Autodesk Inventor part; units mm, degrees
ref_plane "YZ Plane" through (0, 0, 0) normal (1, 0, 0) x (0, 1, 0)
ref_plane "XZ Plane" through (0, 0, 0) normal (0, 1, 0) x (-1, 0, 0)
ref_plane "XY Plane" through (0, 0, 0) normal (0, 0, 1) x (1, 0, 0)
sketch "Esquisse1" plane through (0, 0, 0) normal (0, 0, 1) x (1, 0, 0)
  circle A0 centre (28.6, 24.9) radius 1.5
  circle A1 centre (28.6, -24.78) radius 1.5
  circle A2 centre (-28.75, 24.9) radius 1.5
  circle A3 centre (-28.75, -24.78) radius 1.5
  line L0 (31.1, 27.4) -> (-31.25, 27.4)
  line L1 (-31.25, 27.4) -> (-31.25, -27.28)
  line L2 (-31.25, -27.28) -> (31.1, -27.28)
  line L3 (31.1, -27.28) -> (31.1, 27.4)
  line L4 (-7.575, 16) -> (-0.075, 16)
  line L5 (-0.075, 16) -> (7.425, 16)
  line L6 (7.425, 16) -> (7.425, 10)
  line L7 (7.425, 10) -> (-0.075, 10)
  line L8 (-0.075, 10) -> (-7.575, 10)
  line L9 (-7.575, 10) -> (-7.575, 16)
  line L10 (-0.075, 37.051) -> (-0.075, -38.1524) construction
  line L11 (34.7968, 0.06) -> (-21.7073, 0.06) construction
  line L12 (-7.575, -15.88) -> (-0.075, -15.88)
  line L13 (-0.075, -15.88) -> (7.425, -15.88)
  line L14 (7.425, -15.88) -> (7.425, -9.88)
  line L15 (7.425, -9.88) -> (-0.075, -9.88)
  line L16 (-0.075, -9.88) -> (-7.575, -9.88)
  line L17 (-7.575, -9.88) -> (-7.575, -15.88)
  line L18 (-0.075, -36.931) -> (-0.075, 38.2724) construction
  point P0 (0, 0)
  point P1 (-0.075, 27.4)
  point P2 (31.1, 0.06)
  dimension "d0" = 7.5
  dimension "d1" = 16
  dimension "d2" = 6
extrude "Extrusion1" add sketch "Esquisse1" along normal blind 6
equation "\"d0\" = 0.5 * L_attache_carte"
equation "\"d2\" = epaisseur"
equation "\"d3\" = epaisseur"
equation "\"epaisseur\" = 6"
equation "\"ecartement\" = 25"
equation "\"dvis\" = 3"
equation "\"largeur\" = 32"
equation "\"L_attache_carte\" = 15"
equation "\"marge_attache_carte\" = 5"
equation "\"L_cubi\" = 81.6"
equation "\"taille_trou\" = 7"
equation "\"L_moteur\" = 28.3"
equation "\"marge_trou\" = 2"
equation "\"largeur_cubi\" = 81.6"
equation "\"H_cubi\" = 81.6"
equation "\"epaisseur_wheel\" = 9"
equation "\"H_nez\" = 25"
equation "\"chanfrein\" = 0.5"
equation "\"H_trou_int\" = 0.2"
equation "\"L_trou_int\" = 1"
equation "\"pos_trou_int_1\" = 0.7"
equation "\"pos_trou_int_2\" = 3"
equation "\"epaisseur_metabois\" = 3"
equation "\"L_metabois\" = 8.2"
equation "\"epaisseur_modules\" = 6"
properties part number "support_card"
Verification items for the finished model (mm, model axes). A direction names the side the tool comes from. Give positions to 0.01 mm unless a question says otherwise; leave off trailing zeros. Write each loop counter-clockwise with the first axis right and the second up, starting at its lowest first coordinate (ties: lowest second). Pieces come first, ordered by that corner, then holes. Notation, with made-up numbers: M 34.25,82 L 67.25,82 A27 cw 67.25,102 Z; hole C 35.5,40 d8. An arc over 180 degrees is marked long. One line per question, with ' | ' between items.
1) Section check C-C on x = 28.6. Enter the section's corners in (y, z), plus the area to 3 significant figures.
Result:
outline: M -27.28,0 L -26.28,0 L -26.28,6 L -27.28,6 Z; M -23.28,0 L 23.4,0 L 23.4,6 L -23.28,6 Z; M 26.4,0 L 27.4,0 L 27.4,6 L 26.4,6 Z | area: 292 mm2
2) Section check B-B on z = 2.45. Enter the section's corners in (x, y) (3 decimals), plus the area to 3 significant figures.
Result:
outline: M -31.25,-27.28 L 31.1,-27.28 L 31.1,27.4 L -31.25,27.4 Z; hole C -28.75,-24.78 d3; hole C -28.75,24.9 d3; hole M -7.575,-15.88 L 7.425,-15.88 L 7.425,-9.88 L -7.575,-9.88 Z; hole M -7.575,10 L 7.425,10 L 7.425,16 L -7.575,16 Z; hole C 28.6,-24.78 d3; hole C 28.6,24.9 d3 | area: 3,200 mm2
3) Thickness scan on line 1 along Y through (x, z) = (-28.75, 4.4); line 2 along Y through (x, z) = (7, 5.45); line 3 along X through (y, z) = (-11, 0.35) (3 decimals). Record the ranges inside material, lowest first. Write a range as [from, to].
Result:
line 1: y = [-27.28, -26.28], [-23.28, 23.4], [26.4, 27.4] | line 2: y = [-27.28, -15.88], [-9.88, 10], [16, 27.4] | line 3: x = [-31.25, -7.575], [7.425, 31.1]
4) Section check A-A on y = 24.9. Enter the section's corners in (x, z).
Result:
outline: M -31.25,0 L -30.25,0 L -30.25,6 L -31.25,6 Z; M -27.25,0 L 27.1,0 L 27.1,6 L -27.25,6 Z; M 30.1,0 L 31.1,0 L 31.1,6 L 30.1,6 Z
5) Gauge pin test, flat ends, axial feed: pin 1 Ø2.5 at (x, y) = (28.6, 24.9) entering from +Z; pin 2 Ø12 at (x, y) = (-16.5, 12) entering from -Z. Record the tip position at first contact, or that the pin passes through.
Result:
pin 1: passes through | pin 2: stops at z = 0
6) Set-up check for faces 5 (the flat face through (0, -15.88, 3)), 6 (the flat face through (-31.25, 0, 3)): record each of +Z, -Z, +X, -X, +Y, -Y from which the full face is reachable in a straight line by a thin tool's end or side.
Result:
face 5: +Z, -Z | face 6: +Z, -Z, -X, +Y, -Y
7) Mould release check, pull along Y, two halves, no side actions. Record for faces 1 (the flat face through (0, 27.4, 3)), 2 (the flat face through (0, -9.88, 3)), 3 (the flat face through (-1, -27.28, 3)), 4 (the flat face through (-1, 0, 6)): released by +Y, released by -Y, zero draft, split by the parting line, or undercut.
Result:
face 1: released by +Y | face 2: undercut | face 3: released by -Y | face 4: zero draft
